The listing builds one solid part. Answer for the finished solid, in the listing's coordinates (mm). A direction names the side the tool comes from. Give positions to 0.01 mm unless a question says otherwise; leave off trailing zeros. Loops run counter-clockwise (first coordinate to the right, second up) from the corner with the lowest first, then second, coordinate; pieces in that order, holes last. Notation, with made-up numbers: (-17.75, 71) - (41.25, 71) arc R19 ccw to (41.25, 100) - close; hole circle Ø2 at (-12.5, 81). An arc over 180 degrees is marked (long way). Write each question's results on one line, items separated by ' | '.
from build123d import *

# Parameters (mm, degrees)
SKETCH1_W           = 20
SKETCH1_H           = 18
BOSS_EXTRUDE1_DEPTH = 20
SKETCH2_W           = 12
SKETCH2_H           = 12
CUT_EXTRUDE1_DEPTH  = 14
SKETCH3_W           = 20
SKETCH3_H           = 5
BOSS_EXTRUDE2_DEPTH = 2
LPATTERN1_COUNT     = 6
LPATTERN1_PITCH     = 22
SKETCH4_W           = 20
SKETCH4_H           = 13
BOSS_EXTRUDE3_DEPTH = 2
SKETCH5_W           = 20
SKETCH5_H           = 18
BOSS_EXTRUDE4_DEPTH = 2
SKETCH6_W           = 122
SKETCH6_H           = 2
CUT_EXTRUDE2_DEPTH  = 2
SKETCH7_W           = 134
SKETCH7_H           = 20
BOSS_EXTRUDE5_DEPTH = 6


with BuildPart() as part:
    # Sketch1 → Boss-Extrude1 (new body)
    with BuildSketch(Plane.XY):
        with Locations((10, 9)):
            Rectangle(SKETCH1_W, SKETCH1_H)
    extrude(amount=BOSS_EXTRUDE1_DEPTH)

    # Sketch2 → Cut-Extrude1 (cut)
    with BuildSketch(Plane.XZ):
        with Locations((10, 10)):
            Rectangle(SKETCH2_W, SKETCH2_H)
    extrude(amount=-CUT_EXTRUDE1_DEPTH, mode=Mode.SUBTRACT)

    # Sketch3 → Boss-Extrude2 (add)
    with BuildSketch(Plane(origin=(20, 0, 0), x_dir=(0, 0, -1), z_dir=(1, 0, 0))):
        with Locations((-10, 2.5)):
            Rectangle(SKETCH3_W, SKETCH3_H)
    extrude(amount=BOSS_EXTRUDE2_DEPTH)


with BuildPart() as lpattern1_1:
    # LPattern1: pattern copy
    add(part.part.moved(Location(Vector(1, 0, 0) * (1 * LPATTERN1_PITCH))))


with BuildPart() as lpattern1_2:
    # LPattern1: pattern copy
    add(part.part.moved(Location(Vector(1, 0, 0) * (2 * LPATTERN1_PITCH))))


with BuildPart() as lpattern1_3:
    # LPattern1: pattern copy
    add(part.part.moved(Location(Vector(1, 0, 0) * (3 * LPATTERN1_PITCH))))


with BuildPart() as lpattern1_4:
    # LPattern1: pattern copy
    add(part.part.moved(Location(Vector(1, 0, 0) * (4 * LPATTERN1_PITCH))))


with BuildPart() as lpattern1_5:
    # LPattern1: pattern copy
    add(part.part.moved(Location(Vector(1, 0, 0) * (5 * LPATTERN1_PITCH))))


with BuildPart() as lpattern1_4_1:
    add(lpattern1_4.part)

    # Combine1: union LPattern1_5, part, LPattern1_1, LPattern1_2, LPattern1_3
    add(lpattern1_5.part)
    add(part.part)
    add(lpattern1_1.part)
    add(lpattern1_2.part)
    add(lpattern1_3.part)

    # Sketch4 → Boss-Extrude3 (add)
    with BuildSketch(Plane(origin=(130, 0, 0), x_dir=(0, 0, -1), z_dir=(1, 0, 0))):
        with Locations((-10, 11.5)):
            Rectangle(SKETCH4_W, SKETCH4_H)
    extrude(amount=BOSS_EXTRUDE3_DEPTH)

    # Sketch5 → Boss-Extrude4 (add)
    with BuildSketch(Plane.ZY):
        with Locations((10, 9)):
            Rectangle(SKETCH5_W, SKETCH5_H)
    extrude(amount=BOSS_EXTRUDE4_DEPTH)

    # Sketch6 → Cut-Extrude2 (cut)
    with BuildSketch(Plane(origin=(0, 0, 0), x_dir=(-1, 0, 0), z_dir=(0, -1, 0))):
        with Locations((-65, -10)):
            Rectangle(SKETCH6_W, SKETCH6_H)
    extrude(amount=-CUT_EXTRUDE2_DEPTH, mode=Mode.SUBTRACT)

    # Sketch7 → Boss-Extrude5 (add)
    with BuildSketch(Plane(origin=(0, 0, 0), x_dir=(-1, 0, 0), z_dir=(0, -1, 0))):
        with Locations((-65, -10)):
            Rectangle(SKETCH7_W, SKETCH7_H)
    extrude(amount=BOSS_EXTRUDE5_DEPTH)


solid = lpattern1_4_1.part
Item 1: Find the intervals of material crossed by line 1 along X through (y, z) = (6.75, 1.5); line 2 along Z through (x, y) = (7.5, 8); line 3 along Y through (x, z) = (57, 12), in increasing order. Write a range as [from, to].
Values found:
line 1: x = [-2, 20], [22, 42], [44, 64], [66, 86], [88, 108], [110, 132] | line 2: z = [0, 4], [16, 20] | line 3: y = [-6, 0], [14, 18]
Item 2: A cutting plane is placed at B-B, the plane y = 15.5. Determine the outline of the cut face in (x, z).
Values found:
outline: (-2, 0) - (20, 0) - (20, 20) - (-2, 20) - close; (22, 0) - (42, 0) - (42, 20) - (22, 20) - close; (44, 0) - (64, 0) - (64, 20) - (44, 20) - close; (66, 0) - (86, 0) - (86, 20) - (66, 20) - close; (88, 0) - (108, 0) - (108, 20) - (88, 20) - close; (110, 0) - (132, 0) - (132, 20) - (110, 20) - close
Item 3: A cutting plane is placed at D-D, the plane z = 14.5. Count the separate pieces of the cut face and the enclosed holes in it, plus the area to 3 significant figures.
Values found:
separate pieces: 1 | enclosed holes: 6 | area: 2,080 mm²
Item 4: For a pull along Z with two mould halves and no side action, classify faces 1 (the face through (120, 7, 16)), 2 (the face through (54, 18, 10)) as released by +Z, released by -Z, zero draft, split by the parting line, or undercut.
Values found:
face 1: undercut | face 2: zero draft
Item 5: A flat-ended cylindrical pin translates along its axis: P1, Ø0.6, axis at x = 43, z = 12.5, coming from the +Y side. Find the tip coordinate at first contact, or state that the pin passes through.
Values found:
P1: stops at y = 5
Item 6: A cutting plane is placed at A-A, the plane x = 72.5. Determine the outline of the cut face in (y, z).
Values found:
outline: (-6, 0) - (18, 0) - (18, 20) - (-6, 20) - close; hole (0, 4) - (14, 4) - (14, 16) - (0, 16) - close
Item 7: A cutting plane is placed at C-C, the plane z = 2. Determine the outline of the cut face in (x, y).
Values found:
outline: (-2, -6) - (132, -6) - (132, 18) - (110, 18) - (110, 5) - (108, 5) - (108, 18) - (88, 18) - (88, 5) - (86, 5) - (86, 18) - (66, 18) - (66, 5) - (64, 5) - (64, 18) - (44, 18) - (44, 5) - (42, 5) - (42, 18) - (22, 18) - (22, 5) - (20, 5) - (20, 18) - (-2, 18) - close
Item 8: For faces 3 (the face through (76, 18, 10)), 4 (the face through (64, 11, 10)), 5 (the face through (48, 7, 10)), determine the directions among +Z, -Z, +X, -X, +Y, -Y from which every point of the face is accessible in a straight line to the end or side of a thin tool.
Values found:
face 3: +Z, -Z, +X, -X, +Y | face 4: +Z, -Z, +Y | face 5: none
